```python
from build123d import *

# Parameters (mm, degrees)
BOSS_EXTRUDE1_DEPTH     = 3.175
F_1_1_115_DOWEL_HOLE1_D = 28.321
F_10_CLEARANCE_HOLE1_D  = 5.1054
FILLET1_R               = 38.1
F_1_1_115_DOWEL_HOLE2_D = 28.321
F_8_CLEARANCE_HOLE_D    = 4.4958
F_1_1_115_DOWEL_HOLE3_D = 28.321


with BuildPart() as part:
    # Sketch1 → Boss-Extrude1 (new body)
    with BuildSketch(Plane(origin=(0, 0, 0), x_dir=(1, 0, 0), z_dir=(0, 1, 0))):
        with BuildLine():
            Line((-123.825, -57.15), (123.825, -57.15))
            Line((123.825, -57.15), (123.825, 57.15))
            Line((123.825, 57.15), (52.74706153, 57.15))
            ThreePointArc((52.74706153, 57.15), (0, 38.1), (-52.74706153, 57.15))
            Line((-52.74706153, 57.15), (-123.825, 57.15))
            Line((-123.825, 57.15), (-123.825, -57.15))
        make_face()
    extrude(amount=BOSS_EXTRUDE1_DEPTH)

    # 1 (1.115) Dowel Hole1 (through all)
    with Locations(Plane(origin=(0, 3.175, 0), x_dir=(1, 0, 0), z_dir=(0, 1, 0))):
        with Locations((19.05, -23.906942448)):
            Hole(F_1_1_115_DOWEL_HOLE1_D / 2)

    # #10 Clearance Hole1 (through all)
    with Locations(Plane(origin=(0, 3.175, 0), x_dir=(1, 0, 0), z_dir=(0, 1, 0))):
        with Locations((1.55, -41.406942448), (36.55, -6.406942448), (1.089487758, -5.946430205), (37.010512242, -41.86745469)):
            Hole(F_10_CLEARANCE_HOLE1_D / 2)

    # Fillet1
    fillet1_edges = [part.edges().sort_by_distance(p)[0] for p in [
        (-123.825, 1.5875, -57.15),
        (-123.825, 1.5875, 57.15),
        (123.825, 1.5875, 57.15),
        (123.825, 1.5875, -57.15),
    ]]
    fillet(fillet1_edges, radius=FILLET1_R)

    # 1 (1.115) Dowel Hole2 (through all)
    with Locations(Plane(origin=(0, -34.925, 0), x_dir=(-1, 0, 0), z_dir=(0, -1, 0))):
        with Locations((82.55, 28.448), (-82.55, 28.448)):
            Hole(F_1_1_115_DOWEL_HOLE2_D / 2)

    # #8 Clearance Hole (through all)
    with Locations(Plane(origin=(0, 3.175, 0), x_dir=(1, 0, 0), z_dir=(0, 1, 0))):
        with Locations((-98.425, -6.35), (-60.325, -31.75), (-47.625, 38.1), (47.625, 38.1), (60.325, -31.75), (98.425, -6.35)):
            Hole(F_8_CLEARANCE_HOLE_D / 2)

    # 1 (1.115) Dowel Hole3 (through all)
    with Locations(Plane(origin=(0, -34.925, 0), x_dir=(-1, 0, 0), z_dir=(0, -1, 0))):
        with Locations((19.05, -23.906942448)):
            Hole(F_1_1_115_DOWEL_HOLE3_D / 2)


solid = part.part
```
Design review of the part built by this model. Coordinates are the model's own, in mm. Coordinates: 2 decimals unless noted, no trailing zeros. Order: outer loops, then holes, each group sorted by start corner. A loop starts at its lowest first (then second) coordinate and runs counter-clockwise, first axis right, second up.
1) Clearance check with a flat-ended pin moving along its axis: pin 1 (6 mm diameter, centred on x = 1.55, z = 41.41, fed in from -Y). State where the tip first meets the part, or that it passes through.
2) Take a section at C-C, the plane x = 19. Give the boundary of the cut face in (y, z) (3 decimals).
3) Mouldability with a two-part tool opening along Z and no side actions: class faces 1 (the cylindrical face through (1.64, 1.57, 8.44)), 2 (the cylindrical face through (112.96, 1.61, -45.693)), 3 (the cylindrical face through (-112.368, 1.61, 46.285)) as +Z half, -Z half, draft (parallel to the pull), parting line (faces both ways), or undercut.
4) Take a section at B-B, the plane y = 2.3. State how many separate pieces and enclosed holes the cut face has, and give its area (3 significant figures).
5) Wall thickness on line 1 along Z through (x, y) = (1.55, 1); line 2 along X through (y, z) = (1.5, -17) (3 decimals); line 3 along X through (y, z) = (1.75, 5.5) (3 decimals): over which ranges is each line inside the solid? List them lowest first.
Returned:
1. pin 1: stops at y = 0
2. outline: (0, -40.316) - (3.175, -40.316) - (3.175, 9.747) - (0, 9.747) - close; (0, 38.067) - (3.175, 38.067) - (3.175, 57.15) - (0, 57.15) - close
3. face 1: undercut
3. face 2: -Z half
3. face 3: +Z half
4. separate pieces: 1
4. enclosed holes: 14
4. area: 23,000 mm2
5. line 1: z = -38.11 to 3.44, 8.46 to 38.85, 43.96 to 57.15
5. line 2: x = -123.825 to -90.884, -74.216 to 74.216, 90.884 to 123.825
5. line 3: x = -123.825 to -100.506, -96.344 to -1.424, 3.603 to 34.164, 38.936 to 96.344, 100.506 to 123.825
